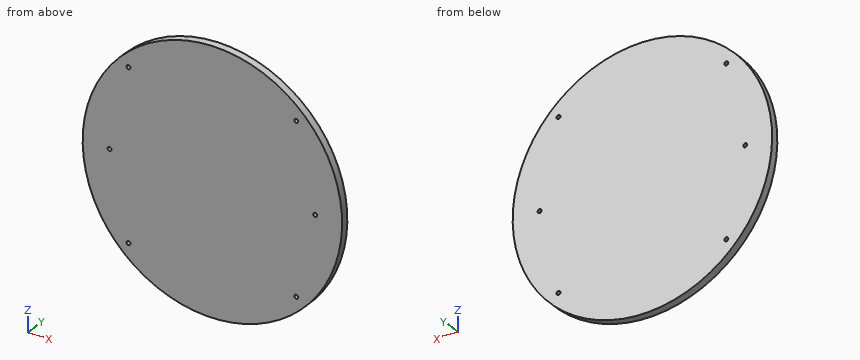
from build123d import *

# Parameters (mm, degrees)
SKETCH1_R           = 82
BOSS_EXTRUDE1_DEPTH = 5
SKETCH14_R          = 1.25
CUT_EXTRUDE2_DEPTH  = 133
SKETCH15_R          = 1.25
CUT_EXTRUDE3_DEPTH  = 10
CIRPATTERN1_COUNT   = 2


with BuildPart() as part:
    # Sketch1 → Boss-Extrude1 (new body)
    with BuildSketch(Plane(origin=(0, 0, 0), x_dir=(1, 0, 0), z_dir=(0, 1, 0))):
        with Locations(Location((0, 0, 0), (0, 0, 270))):
            Circle(SKETCH1_R)
    extrude(amount=BOSS_EXTRUDE1_DEPTH)

    # Sketch14 → Cut-Extrude2 (cut)
    with BuildSketch(Plane(origin=(0, 5, 0), x_dir=(1, 0, 0), z_dir=(0, 1, 0))):
        with Locations(Location((-53.033008589, 53.033008589, 0), (0, 0, 270))):
            Circle(SKETCH14_R)
        with Locations(Location((53.033008589, 53.033008589, 0), (0, 0, 270))):
            Circle(SKETCH14_R)
        with Locations(Location((53.033008589, -53.033008589, 0), (0, 0, 270))):
            Circle(SKETCH14_R)
        with Locations(Location((-53.033008589, -53.033008589, 0), (0, 0, 270))):
            Circle(SKETCH14_R)
    extrude(amount=-CUT_EXTRUDE2_DEPTH, mode=Mode.SUBTRACT)

    # Sketch15 → Cut-Extrude3 (cut)
    with BuildSketch(Plane(origin=(0, 5, 0), x_dir=(1, 0, 0), z_dir=(0, 1, 0))):
        with Locations(Location((-65, 0, 0), (0, 0, 270))):
            Circle(SKETCH15_R)
    cut_extrude3 = extrude(amount=-CUT_EXTRUDE3_DEPTH, mode=Mode.SUBTRACT)

    # CirPattern1: Cut-Extrude3 ×2 about axis
    cirpattern1_axis = Axis((0, 0, 0), (0, 1, 0))
    for i in range(1, CIRPATTERN1_COUNT):
        add(cut_extrude3.rotate(cirpattern1_axis, i * 360 / CIRPATTERN1_COUNT), mode=Mode.SUBTRACT)


solid = part.part
The model under review builds one solid part; all positions refer to its coordinate system, in mm. Coordinates: 2 decimals unless noted, no trailing zeros. Write each loop counter-clockwise with the first axis right and the second up, starting at its lowest first coordinate (ties: lowest second). Pieces come first, ordered by that corner, then holes. Notation, with made-up numbers: (42, 41) - (59, 41) arc R32 ccw to (59, 76) - close; hole circle Ø4 at (62, -28). An arc over 180 degrees is marked (long way). Answer as a JSON object with one key per item and string values. Group by question number.
1. Clearance check with flat-ended pins moving along their axes: pin 1 Ø1 at (x, y) = (43, 1) entering from -Z; pin 2 Ø2 at (x, y) = (7, 1) entering from +Z. State where each tip first meets the part, or that it passes through.
2. Add section B-B (x = 48). Give the boundary of the cut face in (y, z), plus the area to 3 significant figures.
3. Add section C-C (z = 36.5). Give the boundary of the cut face in (x, y), plus the area to 3 significant figures.
4. Add section A-A (y = 2.3). Give the boundary of the cut face in (x, z), plus the area to 3 significant figures.
5. To check wall thickness, follow probe 1 along X at (y, z) = (2.95, 0); probe 2 along Z at (x, y) = (53, 3.4); probe 3 along Z at (x, y) = (-65, 1.1). State the ranges of each line that lie inside material, in increasing order.
Findings:
{
 "1": {"pin 1": "z = -70.13", "pin 2": "z = 81.78"},
 "2": {"outline": "(0, -66.48) - (5, -66.48) - (5, 66.48) - (0, 66.48) - close", "area": "665 mm²"},
 "3": {"outline": "(-73.43, 0) - (73.43, 0) - (73.43, 5) - (-73.43, 5) - close", "area": "734 mm²"},
 "4": {"outline": "circle Ø164 at (0, 0); hole circle Ø2.5 at (-65, 0); hole circle Ø2.5 at (-53.03, -53.03); hole circle Ø2.5 at (-53.03, 53.03); hole circle Ø2.5 at (53.03, -53.03); hole circle Ø2.5 at (53.03, 53.03); hole circle Ø2.5 at (65, 0)", "area": "21,100 mm²"},
 "5": {"probe 1": "-82 to -66.25, -63.75 to 63.75, 66.25 to 82", "probe 2": "-62.57 to -54.28, -51.78 to 51.78, 54.28 to 62.57", "probe 3": "-49.99 to -1.25, 1.25 to 49.99"}
}
